For this review, take the finished solid that the model builds, in its own axes (mm). A direction names the side the tool comes from. Coordinates: 2 decimals unless noted, no trailing zeros. Write each loop counter-clockwise with the first axis right and the second up, starting at its lowest first coordinate (ties: lowest second). Pieces come first, ordered by that corner, then holes. Notation, with made-up numbers: (33, 71) -> (54, 71) arc R21 ccw to (54, 98) -> close; hole circle Ø3 at (76, 14). An arc over 180 degrees is marked (long way). Put each result on its own line as item: value. Start each with the question number.
Item 1: Consider section B-B on z = 0. Give the number of separate pieces and of enclosed holes in the cut face, and give its area (3 significant figures).
Item 2: Consider section A-A on x = 76.2. Give the boundary of the cut face in (y, z) (3 decimals).
Item 3: For faces 1 (the flat face through (0.5, 35.2, 38.1)), 2 (the flat face through (98.425, -10, 1)), 3 (the flat face through (-83, 12.7, 9)), list the 3-axis set-ups (+Z, -Z, +X, -X, +Y, -Y) from which the entire face can be reached by the end or side of a thin tool; tool diameter is ignored.
Item 4: Insertion check: P1, Ø12, axis at y = 31.5, z = 30.5, coming from the -X side; P2, Ø2, axis at x = -14.5, z = -21.5, coming from the -Y side; P3, Ø14.5, axis at x = 66, z = 3, coming from the +Y side. Each pin has a flat end and moves straight along its axis. Give the tip position at first contact, or say it passes through.
Item 5: To check wall thickness, follow L1, parallel to Z at x = -76, y = 9; L2, parallel to Y at x = 95.5, z = -26; L3, parallel to X at y = 5.5, z = -15. State the ranges of each line that lie inside material, in increasing order.
Item 6: Consider section D-D on x = 0. Give the boundary of the cut face in (y, z), and give its area (3 significant figures).
Item 7: The part is to be moulded in two halves that separate along X. For faces 4 (the cylindrical face through (-0.783, 47.746, 0.516)), 5 (the flat face through (60, 0, 1)), 6 (the flat face through (-104, -19.05, 0)), say which applies: +X half, -X half, draft (parallel to the pull), parting line (faces both ways), or undercut.
```python
from build123d import *

# Parameters (mm, degrees)
BOSS_EXTRUDE1_DEPTH = 38.1
SKETCH3_R           = 9.525
CUT_EXTRUDE1_DEPTH  = 123.592896731
FILLET1_R           = 9.652
FILLET2_R           = 1.27


with BuildPart() as part:
    # Sketch1 → Boss-Extrude1 (new, symmetric)
    with BuildSketch(Plane.XY):
        with BuildLine():
            Line((-35.052, 0), (-98.425, 0))
            Line((-98.425, 0), (-98.425, -19.05))
            Line((-98.425, -19.05), (-111.125, -19.05))
            Line((-111.125, -19.05), (-111.125, 12.7))
            Line((-111.125, 12.7), (-46.032200729, 12.7))
            ThreePointArc((-46.032200729, 12.7), (0, 47.752), (46.032200729, 12.7))
            Line((46.032200729, 12.7), (111.125, 12.7))
            Line((111.125, 12.7), (111.125, -19.05))
            Line((111.125, -19.05), (98.425, -19.05))
            Line((98.425, -19.05), (98.425, 0))
            Line((98.425, 0), (35.052, 0))
            ThreePointArc((35.052, 0), (0, 35.052), (-35.052, 0))
        make_face()
    extrude(amount=BOSS_EXTRUDE1_DEPTH, both=True)

    # Sketch3 → Cut-Extrude1 (cut, through all)
    with BuildSketch(Plane(origin=(0, 12.7, 0), x_dir=(1, 0, 0), z_dir=(0, 1, 0))):
        with Locations(Location((-76.2, 0, 0), (0, 0, 180))):
            Circle(SKETCH3_R)
        with Locations(Location((76.2, 0, 0), (0, 0, 180))):
            Circle(SKETCH3_R)
    extrude(amount=-CUT_EXTRUDE1_DEPTH, mode=Mode.SUBTRACT)

    # Fillet1
    fillet1_edges = [part.edges().sort_by_distance(p)[0] for p in [
        (-104.775, -19.05, -38.1),
        (104.775, -19.05, -38.1),
        (104.775, -19.05, 38.1),
        (-111.125, 12.7, 0),
        (-46.032200729, 12.7, 0),
        (46.032200729, 12.7, 0),
        (111.125, 12.7, 0),
        (-104.775, -19.05, 38.1),
    ]]
    fillet(fillet1_edges, radius=FILLET1_R)

    # Fillet2
    fillet2_edges = [part.edges().sort_by_distance(p)[0] for p in [
        (111.125, -19.05, 0),
        (111.125, -3.175, -38.1),
        (111.125, -3.175, 38.1),
        (111.125, -16.222994652, 35.272994652),
        (111.125, -16.222994652, -35.272994652),
        (-111.125, -3.175, -38.1),
        (-77.173251465, 12.7, -38.1),
        (0, 47.752, -38.1),
        (77.173251465, 12.7, -38.1),
        (108.297994652, 9.872994652, -38.1),
        (-108.297994652, 9.872994652, -38.1),
        (-111.125, -19.05, 0),
        (-111.125, -3.175, 38.1),
        (-111.125, -16.222994652, 35.272994652),
        (-111.125, -16.222994652, -35.272994652),
        (-77.173251465, 12.7, 38.1),
        (0, 47.752, 38.1),
        (77.173251465, 12.7, 38.1),
        (108.297994652, 9.872994652, 38.1),
        (-108.297994652, 9.872994652, 38.1),
        (-47.540305771, 14.307243194, -38.1),
        (-47.540305771, 14.307243194, 38.1),
        (47.540305771, 14.307243194, -38.1),
        (47.540305771, 14.307243194, 38.1),
    ]]
    fillet(fillet2_edges, radius=FILLET2_R)


solid = part.part
```
Return value:
1. separate pieces: 3
1. enclosed holes: 0
1. area: 3,250 mm^2
2. outline: (0, -38.1) -> (11.43, -38.1) arc R1.27 ccw to (12.7, -36.83) -> (12.7, -9.525) -> (0, -9.525) -> close; (0, 9.525) -> (12.7, 9.525) -> (12.7, 36.83) arc R1.27 ccw to (11.43, 38.1) -> (0, 38.1) -> close
3. face 1: +Z, +X, -X, +Y, -Y
3. face 2: +Z, -Z, -Y
3. face 3: +Z, -Z, -X, +Y
4. P1: x = -40.37
4. P2: y = 31.44
4. P3: y = 12.7
5. L1: -38.1 to -9.52, 9.52 to 38.1
5. L2: 0 to 12.7
5. L3: -110.81 to -34.62, 34.62 to 110.81
6. outline: (35.05, -38.1) -> (46.48, -38.1) arc R1.27 ccw to (47.75, -36.83) -> (47.75, 36.83) arc R1.27 ccw to (46.48, 38.1) -> (35.05, 38.1) -> close
6. area: 967 mm^2
7. face 4: parting line
7. face 5: undercut
7. face 6: draft
